from build123d import *

# Parameters (mm, degrees)
BOSS_EXTRUDE1_DEPTH = 3.175
SKETCH2_W           = 1.5875
SKETCH2_H           = 1.5875
CUT_EXTRUDE1_DEPTH  = 3.175


with BuildPart() as part:
    # Sketch1 → Boss-Extrude1 (new body)
    with BuildSketch(Plane.XY):
        with BuildLine():
            Line((-24.470793716, 23.241427561), (-24.482874985, 13.608728252))
            Line((-24.482874985, 13.608728252), (19.967125015, -5.441271748))
            ThreePointArc((19.967125015, -5.441271748), (18.373232421, -7.022379153), (19.954339827, -8.616271748))
            Line((19.954339827, -8.616271748), (27.492125015, -8.616271748))
            ThreePointArc((27.492125015, -8.616271748), (28.097157471, -8.173526248), (27.858189288, -7.462905352))
            Line((27.858189288, -7.462905352), (2.504625015, 10.433728252))
            Line((2.504625015, 10.433728252), (-13.370374985, 13.608728252))
            Line((-13.370374985, 13.608728252), (-13.370374985, 23.133728252))
            Line((-13.370374985, 23.133728252), (-24.470793716, 23.241427561))
        make_face()
    extrude(amount=BOSS_EXTRUDE1_DEPTH)

    # Sketch2 → Cut-Extrude1 (cut)
    with BuildSketch(Plane.XY.offset(3.175)):
        with Locations((-14.164124985, 20.752478252)):
            Rectangle(SKETCH2_W, SKETCH2_H)
    extrude(amount=-CUT_EXTRUDE1_DEPTH, mode=Mode.SUBTRACT)


solid = part.part
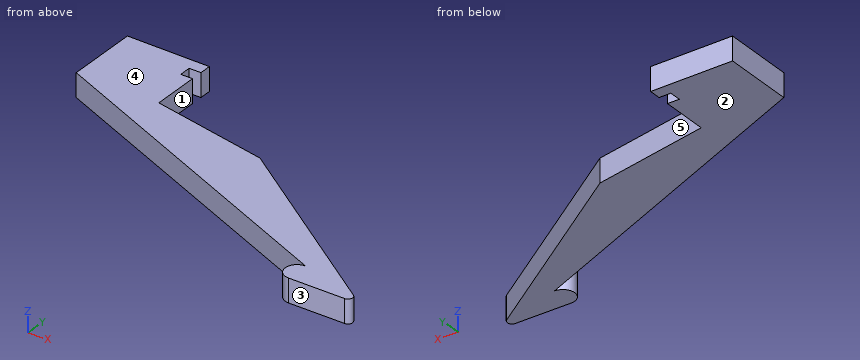
Design review of the part built by this model. Coordinates are the model's own, in mm. Face numbers are marked on the shaded views. A direction names the side the tool comes from. Round coordinates to 2 decimals unless told otherwise and drop trailing zeros. Write each loop counter-clockwise with the first axis right and the second up, starting at its lowest first coordinate (ties: lowest second). Pieces come first, ordered by that corner, then holes.
Item 1: For pin 1 Ø10 at (x, y) = (11, 14) entering from +Z; pin 2 Ø1.5 at (x, y) = (13.5, 3) entering from -Z; pin 3 Ø0.8 at (x, z) = (-14, 1) entering from -Y; pin 4 Ø1 at (y, z) = (18, 2) entering from +X, all flat-tipped, find the tip position at first contact; note any pin that passes through.
Item 2: Consider section C-C on y = 6.5. Give the boundary of the cut face in (x, z) (3 decimals), and give its area (3 significant figures).
Item 3: Consider section D-D on x = -2.5. Give the boundary of the cut face in (y, z) (1 decimal), and give its area (3 significant figures).
Item 4: Consider section A-A on z = 2.4. Give the boundary of the cut face in (x, y), and give its area (3 significant figures).
Item 5: For the marked faces 1 and 2, list the 3-axis set-ups (+Z, -Z, +X, -X, +Y, -Y) from which the entire face can be reached by the end or side of a thin tool; tool diameter is ignored.
Item 6: Wall thickness on L1, parallel to X at y = 16.5, z = 1.7; L2, parallel to X at y = 21, z = 1.65; L3, parallel to Y at x = -2, z = 1.7: over which ranges is each line inside the solid? List them lowest first.
Item 7: Consider section B-B on x = -14. Give the boundary of the cut face in (y, z) (3 decimals).
Item 8: Draft analysis for pull direction Y (two halves, no side actions). For the marked faces 3, 4 and 5, state which applies: released by +Y, released by -Y, zero draft, split by the parting line, or undercut.
Check values:
1. pin 1: passes through
1. pin 2: stops at z = 0
1. pin 3: stops at y = 8.94
1. pin 4: stops at x = -13.37
2. outline: (-7.896, 0) - (8.077, 0) - (8.077, 3.175) - (-7.896, 3.175) - close
2. area: 50.7 mm2
3. outline: (4.2, 0) - (11.4, 0) - (11.4, 3.2) - (4.2, 3.2) - close
3. area: 23.0 mm2
4. outline: (-24.48, 13.61) - (19.97, -5.44) arc R1.59 ccw to (19.95, -8.62) - (27.49, -8.62) arc R0.63 ccw to (27.86, -7.46) - (2.5, 10.43) - (-13.37, 13.61) - (-13.37, 19.96) - (-14.96, 19.96) - (-14.96, 21.55) - (-13.37, 21.55) - (-13.37, 23.13) - (-24.47, 23.24) - close
4. area: 374 mm2
5. face 1: +Z, -Z, +X, +Y
5. face 2: -Z, +X, -X, +Y, -Y
6. L1: x = -24.48 to -13.37
6. L2: x = -24.47 to -14.96
6. L3: y = 3.97 to 11.33
7. outline: (9.116, 0) - (19.959, 0) - (19.959, 3.175) - (9.116, 3.175) - close; (21.546, 0) - (23.14, 0) - (23.14, 3.175) - (21.546, 3.175) - close
8. face 3: released by -Y
8. face 4: zero draft
8. face 5: released by +Y
